Input: part model. Units: mm. Frame: model coordinates. A direction names the side the tool comes from. Give positions to 0.01 mm unless a question says otherwise; leave off trailing zeros. Loops run counter-clockwise (first coordinate to the right, second up) from the corner with the lowest first, then second, coordinate; pieces in that order, holes last. Notation, with made-up numbers: M 14,-20 L 47,-20 A20 ccw 47,11 Z; hole C 78.5,50.5 d3. An arc over 180 degrees is marked long. Use CSV: the item, a comma, the result in double quotes. Start each with the question number.
Q1. Section C-C, the plane x = -6.5. Output: boundary loops of the cut face in (y, z).
Q2. Section B-B, the plane y = -0.6. Output: boundary loops of the cut face in (x, z).
Q3. Section D-D, the plane x = -16. Output: boundary loops of the cut face in (y, z).
Q4. Material intervals for line 1 along X through (y, z) = (2.2, 0.1); line 2 along Z through (x, y) = (8.5, 0.75); line 3 along Y through (x, z) = (3, -1.8), sorted ascending.
Q5. Pin query (flat end, axial travel): pin 1 (3.5 mm diameter, centred on x = -16.5, z = 1, fed in from -Y); pin 2 (3.5 mm diameter, centred on x = -18.5, y = 0.5, fed in from -Z); pin 3 (1.3 mm diameter, centred on x = 16.5, y = -0.5, fed in from +Z). Return the tip coordinate at first contact, or that it passes through.
Q6. Section A-A, the plane z = 0. Output: boundary loops of the cut face in (x, y).
Q7. Reachability of faces 1 (the flat face through (17, 2.123, 0)), 2 (the flat face through (15, -2.5, 0)), 3 (the flat face through (17, 0, -2.12)) from +Z, -Z, +X, -X, +Y, -Y: full face, straight path, thin tool, end or side. Return the list, or none.
from build123d import *

# Parameters (mm, degrees)
SKETCH1_R           = 3
BOSS_EXTRUDE1_DEPTH = 15
SKETCH2_W           = 4.24
SKETCH2_H           = 4.245279732
BOSS_EXTRUDE2_DEPTH = 5


with BuildPart() as part:
    # Sketch1 → Boss-Extrude1 (new body)
    with BuildSketch(Plane(origin=(0, 0, 0), x_dir=(0, 0, -1), z_dir=(1, 0, 0))):
        Circle(SKETCH1_R)
    boss_extrude1 = extrude(amount=BOSS_EXTRUDE1_DEPTH)

    # Sketch2 → Boss-Extrude2 (add)
    with BuildSketch(Plane(origin=(15, 0, 0), x_dir=(0, 0, -1), z_dir=(1, 0, 0))):
        Rectangle(SKETCH2_W, SKETCH2_H)
    boss_extrude2 = extrude(amount=BOSS_EXTRUDE2_DEPTH)

    # Mirror1: Boss-Extrude1, Boss-Extrude2 across plane
    add(boss_extrude1.mirror(Plane(origin=(0, 0, 0), x_dir=(0, 0, 1), z_dir=(1, 0, 0))))
    add(boss_extrude2.mirror(Plane(origin=(0, 0, 0), x_dir=(0, 0, 1), z_dir=(1, 0, 0))))


solid = part.part
A:
1,outline,"C 0,0 d6"
2,outline,"M -20,-2.12 L -15,-2.12 L -15,-2.94 L 15,-2.94 L 15,-2.12 L 20,-2.12 L 20,2.12 L 15,2.12 L 15,2.94 L -15,2.94 L -15,2.12 L -20,2.12 Z"
3,outline,"M -2.12,-2.12 L 2.12,-2.12 L 2.12,2.12 L -2.12,2.12 Z"
4,line 1,"-15 to 15"
4,line 2,"-2.9 to 2.9"
4,line 3,"-2.4 to 2.4"
5,pin 1,"y = -3"
5,pin 2,"z = -2.12"
5,pin 3,"z = 2.12"
6,outline,"M -20,-2.12 L -15,-2.12 L -15,-3 L 15,-3 L 15,-2.12 L 20,-2.12 L 20,2.12 L 15,2.12 L 15,3 L -15,3 L -15,2.12 L -20,2.12 Z"
7,face 1,"+Z, -Z, +X, +Y"
7,face 2,"+Z, -Z, +X, -Y"
7,face 3,"-Z, +X, +Y, -Y"
